```python
from build123d import *

# Parameters (mm, degrees)
F0_R     = 22.545516
F1_DEPTH = 25.4
F3_D     = 9
F4_R     = 3


with BuildPart() as f1:
    # F0 (on Top) → F1 (new body)
    with BuildSketch(Plane.XY):
        with Locations((-23.601482, 23.307687)):
            Circle(F0_R)
    extrude(amount=F1_DEPTH)

    # F3 (through all)
    with Locations(Plane.XZ):
        with Locations((-28.820381, 16.578948)):
            Hole(F3_D / 2)

    # F4
    f4_edges = [f1.edges().sort_by_distance(p)[0] for p in [
        (-46.146997, 23.307687, 25.4),
        (-46.146997, 23.307687, 0),
    ]]
    fillet(f4_edges, radius=F4_R)


solid = f1.part
```
CAD build for the part. Positions are in the model's coordinates, mm. Coordinates: 2 decimals unless noted, no trailing zeros. Loops run counter-clockwise (first coordinate to the right, second up) from the corner with the lowest first, then second, coordinate; pieces in that order, holes last. Notation, with made-up numbers: (5.5, -30) - (31.5, -30) arc R15 cw to (31.5, -2) - close; hole circle Ø5 at (71, 48.25). An arc over 180 degrees is marked (long way). Use CSV: the item, a comma, the result in double quotes. Start each with the question number.
Q1. Cut at C-C, the plane z = 23. List the corners of the cut face in (x, y).
Q2. Probe probe 1 along Y at (x, z) = (-23, 7.25); probe 2 along X at (y, z) = (9.5, 12.5); probe 3 along Z at (x, y) = (-27.5, 39). List the from-to ranges inside material, lowest first. Write a range as from..to.
Q3. Cut at B-B, the plane z = 16. List the corners of the cut face in (x, y), then the cut area to 3 significant figures.
Q4. Cut at A-A, the plane z = 18.75. List the corners of the cut face in (x, y), then the cut area to 3 significant figures.
Q5. Cut at D-D, the plane z = 8.75. List the corners of the cut face in (x, y).
Q6. Drop flat-ended pins along their axis: P1, Ø8, axis at y = 6, z = 18.5, coming from the -X side; P2, Ø1, axis at x = -13, y = 6.5, coming from the +Z side; P3, Ø6, axis at y = 14, z = 14, coming from the +X side; P4, Ø1, axis at x = -19.5, z = 10, coming from the +Y side. Give the stop position or say it passes through.
Q7. Two-plate mould, pull along X, no slides. Class faces 1 (the flat face through (-24, 24, 25.4)), 2 (the cylindrical face through (-2.097, 30.08, 12.564)), 3 (the cylindrical face through (-30.9, 23.62, 12.59)): +X half, -X half, draft (parallel to the pull), parting line (faces both ways), or undercut.
Here are the results:
1,outline,"circle Ø44.97 at (-23.6, 23.31)"
2,probe 1,"0.77..45.85"
2,probe 2,"-41.42..-30.72, -26.92..-5.78"
2,probe 3,"0..12.28, 20.88..25.4"
3,outline,"(-33.28, 2.95) - (-33.28, 43.67) arc R22.55 ccw to start; (-24.36, 0.77) arc R22.55 ccw (long way) to (-24.36, 45.84) - close"
3,area,"1,210 mm2"
4,outline,"(-32.76, 2.71) - (-32.76, 43.91) arc R22.55 ccw to start; (-24.88, 0.8) arc R22.55 ccw (long way) to (-24.88, 45.82) - close"
4,area,"1,250 mm2"
5,outline,"circle Ø45.09 at (-23.6, 23.31)"
6,P1,"x = -41.8"
6,P2,"z = 25.4"
6,P3,"x = -1.96"
6,P4,"y = 45.56"
7,face 1,"draft"
7,face 2,"parting line"
7,face 3,"undercut"
